```python
from build123d import *

# Parameters (mm, degrees)
SKETCH1_R                            = 7.9375
BOSS_EXTRUDE1_DEPTH                  = 6.35
F_0_257_DIAMETER_HOLE1_D             = 6.5278
SKETCH1_3_R                          = 7.9375
BOSS_EXTRUDE2_DEPTH                  = 9.525
W_0_386_DIAMETER_HOLE1_D             = 9.8044
FILLET1_R                            = 2
F_25_64_0_39063_DIAMETER_HOLE1_D     = 9.922002
F_25_64_0_39063_DIAMETER_HOLE1_DEPTH = 1.524
BOSS_EXTRUDE3_DEPTH                  = 6.35
BOSS_EXTRUDE3_DEPTH_BACK             = 2.54
SKETCH12_R                           = 6.35
SKETCH12_R_2                         = 3.2639


with BuildPart() as part:
    # Sketch1 → Boss-Extrude1 (new body)
    with BuildSketch(Plane(origin=(0, 0, 0), x_dir=(1, 0, 0), z_dir=(0, 1, 0))):
        with BuildLine():
            ThreePointArc((2.26024053, 17.840513709), (0, 16.529128421), (-2.26024053, 17.840513709))
            Line((-2.26024053, 17.840513709), (-19.602540008, 56.648386542))
            ThreePointArc((-19.602540008, 56.648386542), (-27.954355314, 59.871226792), (-31.229481324, 51.539776269))
            Line((-31.229481324, 51.539776269), (-8.744221986, -0.519156562))
            ThreePointArc((-8.744221986, -0.519156562), (0, -6.267358068), (8.744221986, -0.519156562))
            Line((8.744221986, -0.519156562), (31.229481324, 51.539776269))
            ThreePointArc((31.229481324, 51.539776269), (27.954355314, 59.871226792), (19.602540008, 56.648386542))
            Line((19.602540008, 56.648386542), (2.26024053, 17.840513709))
        make_face()
        with Locations(Location((0, 3.257641932, 0), (0, 0, 270))):
            Circle(SKETCH1_R, mode=Mode.SUBTRACT)
    extrude(amount=BOSS_EXTRUDE1_DEPTH)

    # F (0.257) Diameter Hole1 (through all)
    with Locations(Plane(origin=(0, 6.35, 0), x_dir=(1, 0, 0), z_dir=(0, 1, 0))):
        with Locations((-25.4, 54.057641932), (25.4, 54.057641932)):
            Hole(F_0_257_DIAMETER_HOLE1_D / 2)

    # Sketch1<3> → Boss-Extrude2 (add)
    with BuildSketch(Plane(origin=(0, 0, 0), x_dir=(1, 0, 0), z_dir=(0, 1, 0))):
        with Locations(Location((0, 3.257641932, 0), (0, 0, 90))):
            Circle(SKETCH1_3_R)
    extrude(amount=BOSS_EXTRUDE2_DEPTH)

    # W (0.386) Diameter Hole1 (through all)
    with Locations(Plane(origin=(0, 9.525, 0), x_dir=(1, 0, 0), z_dir=(0, 1, 0))):
        with Locations((0, 3.257641932)):
            Hole(W_0_386_DIAMETER_HOLE1_D / 2)

    # Fillet1
    fillet1_edges = [part.edges().sort_by_distance(p)[0] for p in [
        (0, 6.35, 4.679858068),
    ]]
    fillet(fillet1_edges, radius=FILLET1_R)

    # 25/64 (0.39063) Diameter Hole1
    with Locations(Plane(origin=(0, 6.35, 0), x_dir=(1, 0, 0), z_dir=(0, 1, 0))):
        with Locations((-25.4, 54.057641932), (25.4, 54.057641932)):
            Hole(F_25_64_0_39063_DIAMETER_HOLE1_D / 2, depth=F_25_64_0_39063_DIAMETER_HOLE1_DEPTH)

    # Sketch12 → Boss-Extrude3 (add, two sides: drawn at the far end of the back side and taken through both)
    # profile 1 of 2: a face of its own
    with BuildSketch(Plane(origin=(0, 6.35, 0), x_dir=(1, 0, 0), z_dir=(0, 1, 0)).offset(-BOSS_EXTRUDE3_DEPTH_BACK)):
        with Locations(Location((25.4, 54.057641932, 0), (0, 0, 155.921287707))):
            Circle(SKETCH12_R)
        with Locations(Location((25.4, 54.057641932, 0), (0, 0, 270))):
            Circle(SKETCH12_R_2, mode=Mode.SUBTRACT)
    # profile 2 of 2: a face of its own
    with BuildSketch(Plane(origin=(0, 6.35, 0), x_dir=(1, 0, 0), z_dir=(0, 1, 0)).offset(-BOSS_EXTRUDE3_DEPTH_BACK)):
        with Locations(Location((-25.4, 54.057641932, 0), (0, 0, 24.078712293))):
            Circle(SKETCH12_R)
        with Locations(Location((-25.4, 54.057641932, 0), (0, 0, 270))):
            Circle(SKETCH12_R_2, mode=Mode.SUBTRACT)
    extrude(amount=BOSS_EXTRUDE3_DEPTH + BOSS_EXTRUDE3_DEPTH_BACK)


solid = part.part
```
Could you check a few things on this model? Use its own coordinates, in mm. A direction names the side the tool comes from. Give positions to 0.01 mm unless a question says otherwise; leave off trailing zeros. Write each loop counter-clockwise with the first axis right and the second up, starting at its lowest first coordinate (ties: lowest second). Pieces come first, ordered by that corner, then holes. Notation, with made-up numbers: (-32, 16) - (-12, 16) arc R25 ccw to (-12, 31) - close; hole circle Ø5 at (34.25, -15.5). An arc over 180 degrees is marked (long way). One line per item, written item: value. Start each with the question number.
Item 1: Imagine slicing it at B-B, the plane y = 10.75. List the corners of the cut face in (x, z) for me.
Item 2: Imagine slicing it at C-C, the plane y = 1. List the corners of the cut face in (x, z) for me (3 decimals), and give its area (3 significant figures).
Item 3: If we mould it in two halves opening along X, with no side actions, what happens to faces 4 (the face through (24, 12.7, -58)), 5 (the face through (7.75, 8.91, -1.54)), 6 (the face through (-10.81, 3.13, -36.97))? For each: +X half, -X half, draft (parallel to the pull), parting line (faces both ways), or undercut.
Item 4: I'm going to push flat-ended pins straight in: pin 1 (1.5 mm diameter, centred on y = 6.5, z = -45, fed in from -X); pin 2 (8 mm diameter, centred on x = -24, z = -32, fed in from +Y); pin 3 (4 mm diameter, centred on x = -25.4, z = -54.06, fed in from -Y); pin 4 (8 mm diameter, centred on x = -3, z = -1, fed in from +Y) (3 decimals). Where does each tip first touch, or does it pass through?
Item 5: Imagine slicing it at A-A, the plane z = -42. List the corners of the cut face in (x, y) for me.
Item 6: Which directions (+Z, -Z, +X, -X, +Y, -Y) give clear straight access to the entire face, cutting with the end or side of a thin tool? Please do faces 1 (the face through (-28.72, 7.67, -59.47)), 2 (the face through (11.053, 3.131, -37.516)), 3 (the face through (-4, 9.525, -7)).
Item 7: Please list where these lines run through material, in increasing order: line 1 (X direction, y = 2, z = -53); line 2 (X direction, y = 3.75, z = -55); line 3 (Y direction, x = 9, z = -16). Write a range as from..to.
Geometry says:
1. outline: circle Ø12.7 at (-25.4, -54.06); circle Ø12.7 at (25.4, -54.06); hole circle Ø6.53 at (-25.4, -54.06); hole circle Ø6.53 at (25.4, -54.06)
2. outline: (-31.229, -51.54) arc R6.35 ccw to (-19.603, -56.648) - (-2.26, -17.841) arc R2.604 cw to (2.26, -17.841) - (19.603, -56.648) arc R6.35 ccw to (31.229, -51.54) - (8.744, 0.519) arc R9.525 ccw to (-8.744, 0.519) - close; hole circle Ø6.528 at (-25.4, -54.058); hole circle Ø9.804 at (0, -3.258); hole circle Ø6.528 at (25.4, -54.058)
2. area: 1,540 mm^2
3. face 4: draft
3. face 5: parting line
3. face 6: undercut
4. pin 1: x = -28.72
4. pin 2: y = 6.35
4. pin 3: through
4. pin 4: y = 9.525
5. outline: (-27.11, 0) - (-13.06, 0) - (-13.06, 6.35) - (-27.11, 6.35) - close; (13.06, 0) - (27.11, 0) - (27.11, 6.35) - (13.06, 6.35) - close
6. face 1: +Y
6. face 2: -Z, +Y, -Y
6. face 3: +Z, -Z, +X, -X, +Y
7. line 1: -31.66..-28.49, -22.31..-17.97, 17.97..22.31, 28.49..31.66
7. line 2: -31.68..-28.52, -22.28..-18.87, 18.87..22.28, 28.52..31.68
7. line 3: 0..6.35
